The model under review builds one solid part; all positions refer to its coordinate system, in mm. A direction names the side the tool comes from. Give positions to 0.01 mm unless a question says otherwise; leave off trailing zeros. Loops run counter-clockwise (first coordinate to the right, second up) from the corner with the lowest first, then second, coordinate; pieces in that order, holes last. Notation, with made-up numbers: (59.5, 52) - (66.5, 52) arc R30 ccw to (66.5, 83) - close; hole circle Ø4 at (87.5, -10.75). An arc over 180 degrees is marked (long way). Answer as a JSON object with one key per item and string values.
from build123d import *

# Parameters (mm, degrees)
SKETCH1_R                               = 114.3
BOSS_EXTRUDE1_DEPTH                     = 5
SKETCH2_R                               = 90
BOSS_EXTRUDE2_DEPTH                     = 5
SKETCH4_R                               = 90
CUT_EXTRUDE2_DEPTH                      = 3.5
F_6_0MM_DOWEL_HOLE1_D                   = 6
F_6_0MM_DOWEL_HOLE1_DEPTH               = 5
CIRPATTERN1_COUNT                       = 12
CBORE_FOR_M8_HEX_HEAD_BOLT2_D           = 10
CBORE_FOR_M8_HEX_HEAD_BOLT2_DEPTH       = 6.5
CBORE_FOR_M8_HEX_HEAD_BOLT2_CBORE_D     = 18.01
CBORE_FOR_M8_HEX_HEAD_BOLT2_CBORE_DEPTH = 5.68
CIRPATTERN2_COUNT                       = 8


with BuildPart() as part:
    # Sketch1 → Boss-Extrude1 (new body)
    with BuildSketch(Plane(origin=(0, 0, 0), x_dir=(1, 0, 0), z_dir=(0, 1, 0))):
        Circle(SKETCH1_R)
    extrude(amount=BOSS_EXTRUDE1_DEPTH)

    # Sketch2 → Boss-Extrude2 (add)
    with BuildSketch(Plane(origin=(0, 5, 0), x_dir=(1, 0, 0), z_dir=(0, 1, 0))):
        Circle(SKETCH2_R)
    extrude(amount=BOSS_EXTRUDE2_DEPTH)

    # Sketch4 → Cut-Extrude2 (cut)
    with BuildSketch(Plane(origin=(0, 0, 0), x_dir=(-1, 0, 0), z_dir=(0, -1, 0))):
        Circle(SKETCH4_R)
    extrude(amount=-CUT_EXTRUDE2_DEPTH, mode=Mode.SUBTRACT)

    # Ø6.0mm Dowel Hole1
    with Locations(Plane(origin=(0, 5, 0), x_dir=(1, 0, 0), z_dir=(0, 1, 0))):
        with Locations((-6.911227035, 101.364663176)):
            f_6_0mm_dowel_hole1 = Hole(F_6_0MM_DOWEL_HOLE1_D / 2, depth=F_6_0MM_DOWEL_HOLE1_DEPTH)

    # CirPattern1: Ø6.0mm Dowel Hole1 ×12 about axis
    cirpattern1_axis = Axis((0, 0, 0), (0, 1, 0))
    for i in range(1, CIRPATTERN1_COUNT):
        add(f_6_0mm_dowel_hole1.rotate(cirpattern1_axis, i * 360 / CIRPATTERN1_COUNT), mode=Mode.SUBTRACT)

    # CBORE for M8 Hex Head Bolt2
    with Locations(Plane(origin=(0, 3.5, 0), x_dir=(-1, 0, 0), z_dir=(0, -1, 0))):
        with Locations((-45.734775632, 65.637872435)):
            cbore_for_m8_hex_head_bolt2 = CounterBoreHole(CBORE_FOR_M8_HEX_HEAD_BOLT2_D / 2, CBORE_FOR_M8_HEX_HEAD_BOLT2_CBORE_D / 2, CBORE_FOR_M8_HEX_HEAD_BOLT2_CBORE_DEPTH, depth=CBORE_FOR_M8_HEX_HEAD_BOLT2_DEPTH)

    # CirPattern2: CBORE for M8 Hex Head Bolt2 ×8 about axis
    cirpattern2_axis = Axis((0, 0, 0), (0, 1, 0))
    for i in range(1, CIRPATTERN2_COUNT):
        add(cbore_for_m8_hex_head_bolt2.rotate(cirpattern2_axis, i * 360 / CIRPATTERN2_COUNT), mode=Mode.SUBTRACT)


solid = part.part
Q1. Consider section B-B, the plane z = 0. State the section outline as (x, y) points.
Results:
{"outline": "(-114.3, 0) - (-90, 0) - (-90, 3.5) - (90, 3.5) - (90, 0) - (114.3, 0) - (114.3, 5) - (90, 5) - (90, 10) - (-90, 10) - (-90, 5) - (-114.3, 5) - close"}
Q2. Clearance check with flat-ended pins moving along their axes: pin 1 Ø5.5 at (x, z) = (-101.36, 6.91) entering from -Y; pin 2 Ø6 at (x, y) = (47.5, 3.5) entering from +Z; pin 3 Ø8 at (x, z) = (6.91, 101.36) entering from +Y; pin 4 Ø14.5 at (x, z) = (-65.64, -45.73) entering from +Y. State where each tip first meets the part, or that it passes through.
Results:
{"pin 1": "passes through", "pin 2": "stops at z = 105.28", "pin 3": "stops at y = 5", "pin 4": "stops at y = 10"}
Q3. Consider section A-A, the plane x = 0. State the section outline as (y, z) points, plus the area to 3 significant figures.
Results:
{"outline": "(0, -114.3) - (5, -114.3) - (5, -90) - (10, -90) - (10, 90) - (5, 90) - (5, 114.3) - (0, 114.3) - (0, 90) - (3.5, 90) - (3.5, -90) - (0, -90) - close", "area": "1,410 mm^2"}
Q4. For faces 4 (the face through (84, 0, -34)), 5 (the face through (-87.75, 6.3, 13.68)), list the 3-axis set-ups (+Z, -Z, +X, -X, +Y, -Y) from which the entire face can be reached by the end or side of a thin tool; tool diameter is ignored.
Results:
{"face 4": "+Z, -Z, +X, -X, -Y", "face 5": "-Y"}
Q5. The part is to be moulded in two halves that separate along X. For faces 1 (the face through (43.796, 2.465, -88.379)), 2 (the face through (-114.19, 2.46, -5.03)), 3 (the face through (-1, 10, -1)), say which applies: +X half, -X half, draft (parallel to the pull), parting line (faces both ways), or undercut.
Results:
{"face 1": "undercut", "face 2": "parting line", "face 3": "draft"}
Q6. To check wall thickness, follow probe 1 along X at (y, z) = (0.85, 0); probe 2 along Z at (x, y) = (71, 9); probe 3 along X at (y, z) = (6.75, -3). State the ranges of each line that lie inside material, in increasing order. Write a range as [from, to].
Results:
{"probe 1": "x = [-114.3, -90], [90, 114.3]", "probe 2": "z = [-55.31, -18.66], [-9.49, 38.5], [52.97, 55.31]", "probe 3": "x = [-89.95, 89.95]"}
